Check sheet for the modelled part. Datum: model origin and axes. Units: mm. A direction names the side the tool comes from. Give positions to 0.01 mm unless a question says otherwise; leave off trailing zeros. Write each loop counter-clockwise with the first axis right and the second up, starting at its lowest first coordinate (ties: lowest second). Pieces come first, ordered by that corner, then holes. Notation, with made-up numbers: (35.5, 1.5) -> (78.5, 1.5) arc R28 ccw to (78.5, 21.5) -> close; hole circle Ø8 at (-29, 39). An arc over 180 degrees is marked (long way). Answer as a JSON object with one key per item and string values.
from build123d import *

# Parameters (mm, degrees)
SKETCH1_R             = 23.55
SKETCH1_R_2           = 14
BOSS_EXTRUDE4_DEPTH   = 10
SKETCH6_R             = 34.4
SKETCH6_R_2           = 23.55
BOSS_EXTRUDE5_DEPTH   = 10
SKETCH8_R             = 5.9563
BOSS_EXTRUDE7_DEPTH   = 14.3
BOSS_EXTRUDE7_2_DEPTH = 14.3
BOSS_EXTRUDE8_DEPTH   = 10
SKETCH10_R            = 25.832365573
SKETCH10_R_2          = 23.55
BOSS_EXTRUDE9_DEPTH   = 10
BOSS_EXTRUDE10_START  = 10
BOSS_EXTRUDE10_DEPTH  = 10
BOSS_EXTRUDE11_DEPTH  = 27.5
FILLET4_R             = 10
FILLET5_R             = 10
BOSS_EXTRUDE13_DEPTH  = 5


with BuildPart() as part:
    # Sketch1 → Boss-Extrude4 (new body)
    with BuildSketch(Plane(origin=(0, 0, 0), x_dir=(1, 0, 0), z_dir=(0, 1, 0))):
        with Locations(Location((0, 0, 0), (0, 0, 270))):
            Circle(SKETCH1_R)
        with Locations(Location((0, 0, 0), (0, 0, 270))):
            Circle(SKETCH1_R_2, mode=Mode.SUBTRACT)
    extrude(amount=BOSS_EXTRUDE4_DEPTH)



with BuildPart() as body_2:
    # Sketch6 → Boss-Extrude5 (new body)
    with BuildSketch(Plane(origin=(0, 10, 0), x_dir=(1, 0, 0), z_dir=(0, 1, 0))):
        with Locations(Location((0, 0, 0), (0, 0, 270))):
            Circle(SKETCH6_R)
        with Locations(Location((0, 0, 0), (0, 0, 270))):
            Circle(SKETCH6_R_2, mode=Mode.SUBTRACT)
    extrude(amount=BOSS_EXTRUDE5_DEPTH)



with BuildPart() as body_3:
    # Sketch8 → Boss-Extrude7 (new body)
    with BuildSketch(Plane(origin=(0, 20, 0), x_dir=(1, 0, 0), z_dir=(0, 1, 0))):
        with BuildLine():
            ThreePointArc((-55.268702708, 14.537801572), (-65.0875, 0), (-55.268702708, -14.537801572))
            ThreePointArc((-55.268702708, -14.537801572), (-42.522384328, -17.885755457), (-29.343880761, -17.952622702))
            ThreePointArc((-29.343880761, -17.952622702), (-34.4, 0), (-29.343880761, 17.952622702))
            ThreePointArc((-29.343880761, 17.952622702), (-42.522384328, 17.885755457), (-55.268702708, 14.537801572))
        make_face()
        with Locations(Location((-49.4157, 0, 0), (0, 0, 270))):
            Circle(SKETCH8_R, mode=Mode.SUBTRACT)
    extrude(amount=BOSS_EXTRUDE7_DEPTH)


with BuildPart() as body_4:
    # Sketch8 → Boss-Extrude7 2 (new body)
    with BuildSketch(Plane(origin=(0, 20, 0), x_dir=(1, 0, 0), z_dir=(0, 1, 0))):
        with BuildLine():
            ThreePointArc((55.268702708, 14.537801572), (42.522384328, 17.885755457), (29.343880761, 17.952622702))
            ThreePointArc((29.343880761, 17.952622702), (34.4, 0), (29.343880761, -17.952622702))
            ThreePointArc((29.343880761, -17.952622702), (42.522384328, -17.885755457), (55.268702708, -14.537801572))
            ThreePointArc((55.268702708, -14.537801572), (65.0875, 0), (55.268702708, 14.537801572))
        make_face()
        with Locations(Location((49.4157, 0, 0), (0, 0, 90))):
            Circle(SKETCH8_R, mode=Mode.SUBTRACT)
    extrude(amount=BOSS_EXTRUDE7_2_DEPTH)


with BuildPart() as body_2_1:
    add(body_2.part)

    add(body_3.part)  # Boss-Extrude8 merges body 3

    add(body_4.part)  # Boss-Extrude8 merges body 4
    # Sketch9 → Boss-Extrude8 (add)
    with BuildSketch(Plane.XZ.offset(-20)):
        with BuildLine():
            Line((-32.994341825, 18.26698083), (-29.343880761, 17.952622702))
            ThreePointArc((-29.343880761, 17.952622702), (-34.4, 0), (-29.343880761, -17.952622702))
            Line((-29.343880761, -17.952622702), (-32.994341825, -18.26698083))
            ThreePointArc((-32.994341825, -18.26698083), (-37.713514569, 0), (-32.994341825, 18.26698083))
        make_face()
        with BuildLine():
            Line((32.994341825, 18.26698083), (29.343880761, 17.952622702))
            ThreePointArc((29.343880761, 17.952622702), (34.4, 0), (29.343880761, -17.952622702))
            Line((29.343880761, -17.952622702), (32.994341825, -18.26698083))
            ThreePointArc((32.994341825, -18.26698083), (37.713514569, 0), (32.994341825, 18.26698083))
        make_face()
    extrude(amount=BOSS_EXTRUDE8_DEPTH)


with BuildPart() as part_1:
    add(part.part)

    add(body_2_1.part)  # Boss-Extrude9 merges body 2
    # Sketch10 → Boss-Extrude9 (add)
    with BuildSketch(Plane.XZ):
        with Locations(Location((0, 0, 0), (0, 0, 270))):
            Circle(SKETCH10_R)
        with Locations(Location((0, 0, 0), (0, 0, 90))):
            Circle(SKETCH10_R_2, mode=Mode.SUBTRACT)
    extrude(amount=-BOSS_EXTRUDE9_DEPTH)

    # Sketch11 → Boss-Extrude10 (add)
    with BuildSketch(Plane.XZ.offset(BOSS_EXTRUDE10_START)):
        with BuildLine():
            Line((-1.769995947, 13.887660507), (-3.265941597, 25.625080225))
            ThreePointArc((-3.265941597, 25.625080225), (-25.832365573, 0), (-3.265941597, -25.625080225))
            Line((-3.265941597, -25.625080225), (-1.769995947, -13.887660507))
            ThreePointArc((-1.769995947, -13.887660507), (-14, 0), (-1.769995947, 13.887660507))
        make_face()
        with BuildLine():
            Line((1.769995947, -13.887660507), (3.265941597, -25.625080225))
            ThreePointArc((3.265941597, -25.625080225), (25.832365573, 0), (3.265941597, 25.625080225))
            Line((3.265941597, 25.625080225), (1.769995947, 13.887660507))
            ThreePointArc((1.769995947, 13.887660507), (14, 0), (1.769995947, -13.887660507))
        make_face()
    extrude(amount=-BOSS_EXTRUDE10_DEPTH)

    # Sketch12 → Boss-Extrude11 (add)
    with BuildSketch(Plane.XZ.offset(10)):
        with BuildLine():
            Line((-1.769995947, 13.887660507), (-2.517968772, 19.756370366))
            ThreePointArc((-2.517968772, 19.756370366), (-19.916182786, 0), (-2.517968772, -19.756370366))
            Line((-2.517968772, -19.756370366), (-1.769995947, -13.887660507))
            Line((-1.769995947, -13.887660507), (-1.649889079, -12.945283544))
            ThreePointArc((-1.649889079, -12.945283544), (-13.05, 0), (-1.649889079, 12.945283544))
            Line((-1.649889079, 12.945283544), (-1.769995947, 13.887660507))
        make_face()
        with BuildLine():
            Line((1.769995947, 13.887660507), (2.517968772, 19.756370366))
            ThreePointArc((2.517968772, 19.756370366), (19.916182786, 0), (2.517968772, -19.756370366))
            Line((2.517968772, -19.756370366), (1.769995947, -13.887660507))
            Line((1.769995947, -13.887660507), (1.649889079, -12.945283544))
            ThreePointArc((1.649889079, -12.945283544), (13.05, 0), (1.649889079, 12.945283544))
            Line((1.649889079, 12.945283544), (1.769995947, 13.887660507))
        make_face()
    extrude(amount=BOSS_EXTRUDE11_DEPTH)

    # Fillet4
    # the kernel refuses this fillet: 10 mm, written as the material it takes off along each edge
    with BuildSketch(Plane(origin=(0, -10, 0), x_dir=(-0.12642828192325106, 0, -0.9919757504747456), z_dir=(0.9919757504747456, 0, -0.12642828192325106))) as fillet4_piece_1:
        with BuildLine():
            CenterArc((23.05, -4.254115654), FILLET4_R, 154.823283059, 25.176716941)
            Line((13.05, -4.254115654), (12.85, -4.254115654))
            Line((12.85, -4.254115654), (12.85, 0))
            Line((12.85, 0), (13.05, 0.2))
            ThreePointArc((13.05, 0.2), (13.525, 0.2), (13.819, 0.085082313))
            Line((13.819, 0.085082313), (14, 0))
        make_face()
    revolve(axis=Axis((0, -10, 0), (0, 1, 0)), revolution_arc=165.473510519, mode=Mode.SUBTRACT)

    # Fillet5
    # the kernel refuses this fillet: 10 mm, written as the material it takes off along each edge
    with BuildSketch(Plane(origin=(0, -10, 0), x_dir=(-0.6360006800114754, 0, -0.7716884961076852), z_dir=(-0.7716884961076852, 0, 0.6360006800114754))) as fillet5_piece_1:
        with BuildLine():
            CenterArc((23.05, 4.254115654), FILLET5_R, 180, 25.176716941)
            Line((13.05, 4.254115654), (12.85, 4.254115654))
            Line((12.85, 4.254115654), (12.85, 0))
            Line((12.85, 0), (13.05, -0.2))
            ThreePointArc((13.05, -0.2), (13.525, -0.2), (13.819, -0.085082313))
            Line((13.819, -0.085082313), (14, 0))
        make_face()
    revolve(axis=Axis((0, -10, 0), (0, -1, 0)), revolution_arc=258.988485214, mode=Mode.SUBTRACT)

    # Sketch14 → Boss-Extrude13 (add)
    with BuildSketch(Plane.XZ.offset(37.5)):
        with BuildLine():
            Line((-1.649889079, 12.945283544), (-2.670219685, 20.950954455))
            ThreePointArc((-2.670219685, 20.950954455), (-21.120430056, 0), (-2.670219685, -20.950954455))
            Line((-2.670219685, -20.950954455), (-1.649889079, -12.945283544))
            ThreePointArc((-1.649889079, -12.945283544), (-13.05, 0), (-1.649889079, 12.945283544))
        make_face()
        with BuildLine():
            Line((2.670219685, -20.950954455), (1.649889079, -12.945283544))
            ThreePointArc((1.649889079, -12.945283544), (13.05, 0), (1.649889079, 12.945283544))
            Line((1.649889079, 12.945283544), (2.670219685, 20.950954455))
            ThreePointArc((2.670219685, 20.950954455), (21.120430056, 0), (2.670219685, -20.950954455))
        make_face()
    extrude(amount=BOSS_EXTRUDE13_DEPTH)


solid = part_1.part
1. Sectioned sample at A-A, the plane x = 0. Enter the section's corners in (y, z).
Determined:
{"outline": "(0, -25.83) -> (10, -25.83) -> (10, -34.4) -> (20, -34.4) -> (20, -23.55) -> (10, -23.55) -> (10, -14) -> (0, -14) -> close; (0, 14) -> (10, 14) -> (10, 23.55) -> (20, 23.55) -> (20, 34.4) -> (10, 34.4) -> (10, 25.83) -> (0, 25.83) -> close"}
2. Access from +Z, -Z, +X, -X, +Y, -Y to the whole of each face (thin tool, end or side, straight path). Record for faces 1 (the face through (0, 0, -21)), 2 (the face through (34.4, 27, -0.3)), 3 (the face through (20.1, -37.5, 0.1)), 4 (the face through (21.116, -39.965, 0.427)).
Determined:
{"face 1": "-Z, -Y", "face 2": "+Y", "face 3": "+X", "face 4": "+X, -Y"}
3. Sectioned sample at C-C, the plane z = 0. State how many separate pieces and enclosed holes the cut face has, plus the area to 3 significant figures.
Determined:
{"separate pieces": "4", "enclosed holes": "0", "area": "1,750 mm^2"}
4. Sectioned sample at B-B, the plane y = -8. Enter the section's corners in (x, z).
Determined:
{"outline": "(-3.27, -25.63) -> (-1.77, -13.89) arc R14 cw to (-1.77, 13.89) -> (-3.27, 25.63) arc R25.83 ccw to start; (1.77, -13.89) -> (3.27, -25.63) arc R25.83 ccw to (3.27, 25.63) -> (1.77, 13.89) arc R14 cw to start"}
5. Sectioned sample at D-D, the plane y = 28.5. Enter the section's corners in (x, z).
Determined:
{"outline": "(-55.27, -14.54) arc R52.48 ccw to (-29.34, -17.95) arc R34.4 cw to (-29.34, 17.95) arc R52.48 ccw to (-55.27, 14.54) arc R15.67 ccw to start; (29.34, -17.95) arc R52.48 ccw to (55.27, -14.54) arc R15.67 ccw to (55.27, 14.54) arc R52.48 ccw to (29.34, 17.95) arc R34.4 cw to start; hole circle Ø11.91 at (-49.42, 0); hole circle Ø11.91 at (49.42, 0)"}
6. Scan lines: L1, parallel to X at y = 17, z = 0; L2, parallel to X at y = 30.5, z = 4; L3, parallel to X at y = -21, z = -7. Record each from-to range of solid material in increasing order. Write a range as [from, to].
Determined:
{"L1": "[-37.71, -23.55], [23.55, 37.71]", "L2": "[-64.57, -53.83], [-45, -34.17], [34.17, 45], [53.83, 64.57]", "L3": "[-18.65, -11.01], [11.01, 18.65]"}
7. Mould release check, pull along X, two halves, no side actions. Record for faces 5 (the face through (-20.1, -37.5, 0.1)), 6 (the face through (-22.5, 20, -8.1)), 7 (the face through (19.912, -23.557, 0.403)): released by +X, released by -X, zero draft, split by the parting line, or undercut.
Determined:
{"face 5": "zero draft", "face 6": "undercut", "face 7": "released by +X"}
8. Go/stop test with flat-tipped pins: P1, Ø6, axis at x = 43.5, z = -4.5, coming from the -Y side; P2, Ø5, axis at x = 40, z = 1, coming from the -Y side; P3, Ø2, axis at y = 5, z = -24, coming from the -X side. Record where each tip stops, or that it passes through.
Determined:
{"P1": "y = 20", "P2": "y = 10", "P3": "x = -11.76"}
